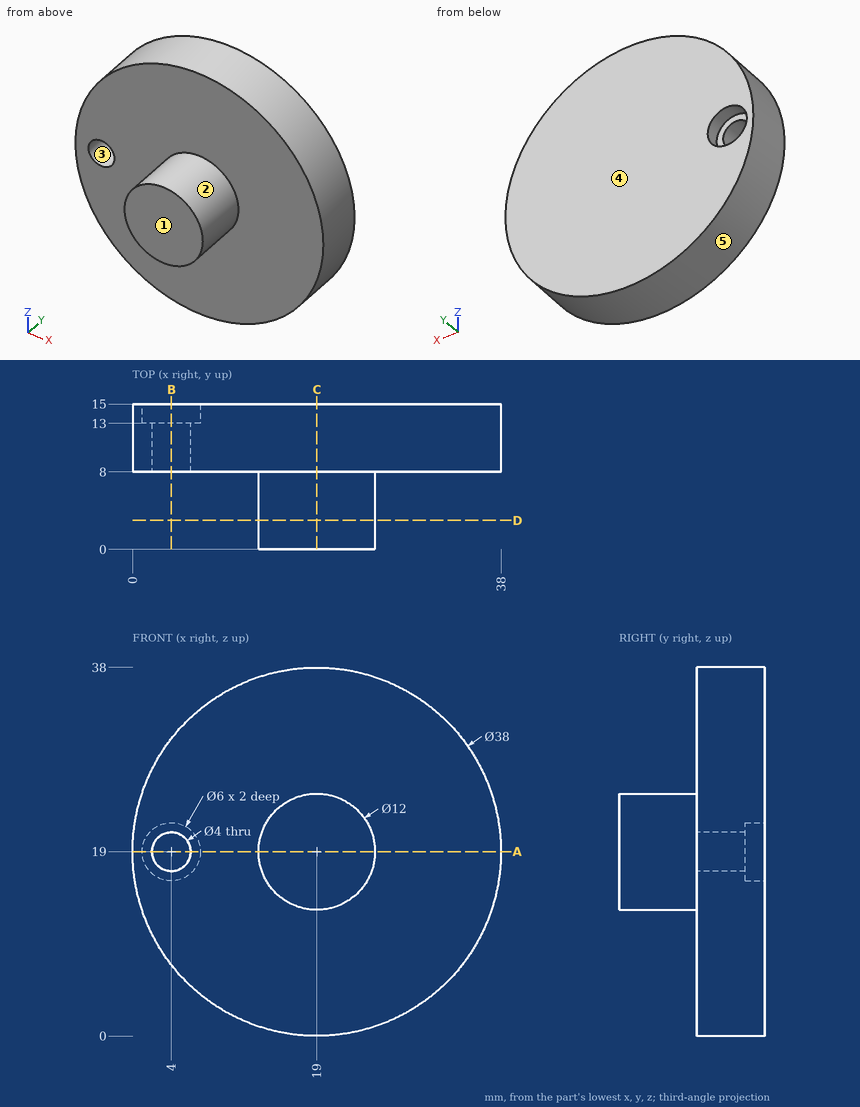
Job drawing, mm, ordinate dimensions from the low corner. One solid piece. A direction names the side the tool comes from. Give positions to 0.01 mm unless a question says otherwise; leave off trailing zeros. Loops run counter-clockwise (first coordinate to the right, second up) from the corner with the lowest first, then second, coordinate; pieces in that order, holes last.
Item 1: Pull direction X, two halves, no side cores. Call the marked faces 3, 4 and 5: released by +X, released by -X, zero draft, split by the parting line, or undercut.
Answers follow:
face 3: undercut
face 4: zero draft
face 5: split by the parting line
Item 2: Slice it at D-D, the plane y = 3. List the corners of the cut face in (x, z).
Answers follow:
outline: circle Ø12 at (19, 19)
Item 3: Flat gauge pins, fed straight in: pin 1 (3 mm diameter, centred on x = 33.5, z = 14, fed in from -Y); pin 2 (4 mm diameter, centred on x = 30, y = 10, fed in from +Z); pin 3 (4 mm diameter, centred on y = 9, z = 13.5, fed in from -X). Where does each tip first touch, or does it go through?
Answers follow:
pin 1: stops at y = 8
pin 2: stops at z = 35.73
pin 3: stops at x = 0.33
Item 4: Which spindle directions (+Z, -Z, +X, -X, +Y, -Y) get a long thin tool onto all of the face, cutting with end or side? Do the marked faces 1 and 2. Say none if no direction does.
Answers follow:
face 1: +Z, -Z, +X, -X, -Y
face 2: -Y
Item 5: Slice it at B-B, the plane x = 4. List the corners of the cut face in (y, z).
Answers follow:
outline: (8, 7.34) - (15, 7.34) - (15, 16) - (13, 16) - (13, 17) - (8, 17) - close; (8, 21) - (13, 21) - (13, 22) - (15, 22) - (15, 30.66) - (8, 30.66) - close
Item 6: Slice it at A-A, the plane z = 19. List the corners of the cut face in (x, y).
Answers follow:
outline: (0, 8) - (2, 8) - (2, 13) - (1, 13) - (1, 15) - (0, 15) - close; (6, 8) - (13, 8) - (13, 0) - (25, 0) - (25, 8) - (38, 8) - (38, 15) - (7, 15) - (7, 13) - (6, 13) - close
Item 7: Slice it at C-C, the plane x = 19. List the corners of the cut face in (y, z), and give its area (3 significant figures).
Answers follow:
outline: (0, 13) - (8, 13) - (8, 0) - (15, 0) - (15, 38) - (8, 38) - (8, 25) - (0, 25) - close
area: 362 mm2
Item 8: Drill centre lines: line 1 (X direction, y = 9.05, z = 19); line 2 (X direction, y = 13.95, z = 19); line 3 (Y direction, x = 20, z = 10). Where is each one in solid material? Low to high.
Answers follow:
line 1: x = 0 to 2, 6 to 38
line 2: x = 0 to 1, 7 to 38
line 3: y = 8 to 15
